Work out the finished part from the listing and answer in its coordinate system (mm). A direction names the side the tool comes from. Give positions to 0.01 mm unless a question says otherwise; leave off trailing zeros. Loops run counter-clockwise (first coordinate to the right, second up) from the corner with the lowest first, then second, coordinate; pieces in that order, holes last. Notation, with made-up numbers: M 51,31 L 67,31 A32 cw 67,67 Z; hole C 88.5,63 d11. An arc over 180 degrees is marked long. Answer in a Markdown table with one row per item. Add a question column.
from build123d import *

# Parameters (mm, degrees)
EXTRUDE_THIN1_DEPTH = 93.98
SKETCH2_W           = 28.622498
SKETCH2_H           = 25.4
BOSS_EXTRUDE1_DEPTH = 5.08


with BuildPart() as part:
    # Sketch1 → Extrude-Thin1 (new body)
    with BuildSketch(Plane.XY):
        Polygon((-18.462498, 59.69), (-18.462498, 62.865), (0, 62.865), (0, 0), (-18.462498, 0), (-18.462498, 3.175), (-23.542498, 3.175), (-23.542498, -5.08), (5.08, -5.08), (5.08, 67.945), (-23.542498, 67.945), (-23.542498, 59.69), align=None)
    extrude(amount=EXTRUDE_THIN1_DEPTH)

    # Sketch2 → Boss-Extrude1 (add)
    with BuildSketch(Plane.XY.offset(93.98)):
        with Locations((-9.231249, 7.62)):
            Rectangle(SKETCH2_W, SKETCH2_H)
    extrude(amount=-BOSS_EXTRUDE1_DEPTH)


solid = part.part
(1) Section A-A, the plane x = -8.25 is taken. Determine the outline of the cut face in (y, z) (3 decimals), and give its area (3 significant figures).
(2) Consider line 1 along X through (y, z) = (2.5, 67); line 2 along Y through (x, z) = (-20.5, 89) (3 decimals); line 3 along Y through (x, z) = (-20, 19) (3 decimals). Determine where each line is inside the solid, lowest interval first. Write a range as from..to.
(3) Which of the six approach directions +Z, -Z, +X, -X, +Y, -Y give full straight-line access (tool end or side, diameter ignored) to faces 5 (the face through (-9, 0, 44)), 6 (the face through (-9, 62.865, 46)), 7 (the face through (-21, 3.175, 44)), 8 (the face through (-12, 20.32, 91))?
(4) Section D-D, the plane y = 19 is taken. Determine the outline of the cut face in (x, z), and give its area (3 significant figures).
(5) Section B-B, the plane z = 52.5 is taken. Determine the outline of the cut face in (x, y) (1 decimal), and give its area (3 significant figures).
(6) Section C-C, the plane x = -20 is taken. Determine the outline of the cut face in (y, z) (3 decimals).
(7) The mould has two halves that part along X. Classify faces 1 (the face through (-6, 16, 93.98)), 2 (the face through (-18.462, 2, 44)), 3 (the face through (-18.462, 61, 46)), 4 (the face through (5.08, 31, 46)): pulls with the +X half, pulls with the -X half, needs draft (parallel to the pull), parting line crosses it, or undercut.
(8) This flat-tipped pin is pushed along its axis until it touches: P1, Ø1.5, axis at y = 32.5, z = 57.5, coming from the -X side. Where does it stop, or does it pass through?
Numbers:
| question | item | result |
|---|---|---|
| 1 | outline | M -5.08,0 L 0,0 L 0,88.9 L 20.32,88.9 L 20.32,93.98 L -5.08,93.98 Z; M 62.865,0 L 67.945,0 L 67.945,93.98 L 62.865,93.98 Z |
| 1 | area | 1,060 mm² |
| 2 | line 1 | x = -23.54..-18.46, 0..5.08 |
| 2 | line 2 | y = -5.08..20.32, 59.69..67.945 |
| 2 | line 3 | y = -5.08..3.175, 59.69..67.945 |
| 3 | face 5 | -Z |
| 3 | face 6 | +Z, -Z |
| 3 | face 7 | -Z, -X |
| 3 | face 8 | +Z, -Z, -X |
| 4 | outline | M -23.54,88.9 L 0,88.9 L 0,0 L 5.08,0 L 5.08,93.98 L -23.54,93.98 Z |
| 4 | area | 597 mm² |
| 5 | outline | M -23.5,-5.1 L 5.1,-5.1 L 5.1,67.9 L -23.5,67.9 L -23.5,59.7 L -18.5,59.7 L -18.5,62.9 L 0,62.9 L 0,0 L -18.5,0 L -18.5,3.2 L -23.5,3.2 Z |
| 5 | area | 642 mm² |
| 6 | outline | M -5.08,0 L 3.175,0 L 3.175,88.9 L 20.32,88.9 L 20.32,93.98 L -5.08,93.98 Z; M 59.69,0 L 67.945,0 L 67.945,93.98 L 59.69,93.98 Z |
| 7 | face 1 | needs draft |
| 7 | face 2 | undercut |
| 7 | face 3 | undercut |
| 7 | face 4 | pulls with the +X half |
| 8 | P1 | stops at x = 0 |
